Read the model definition and answer for the solid it produces. Units are mm, in the model's axes. Round coordinates to 2 decimals unless told otherwise and drop trailing zeros. Write each loop counter-clockwise with the first axis right and the second up, starting at its lowest first coordinate (ties: lowest second). Pieces come first, ordered by that corner, then holes.
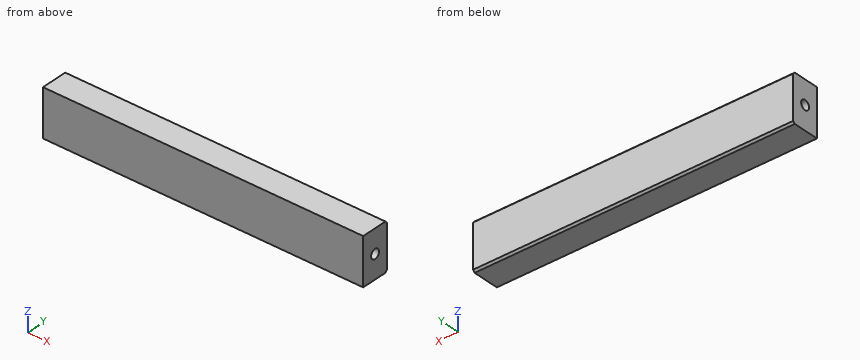
from build123d import *

# Parameters (mm, degrees)
SKETCH_1_W          = 85
SKETCH_1_H          = 7.5
EXTRUDE_1_DEPTH     = 12.5
SKETCH_2_R          = 1.25
CUT_EXTRUDE_1_DEPTH = 86.996002814
CHAMFER_1_SIZE      = 0.5


with BuildPart() as part:
    # 草图1 → 凸台-拉伸1 (new body)
    with BuildSketch(Plane.XY):
        Rectangle(SKETCH_1_W, SKETCH_1_H)
    extrude(amount=EXTRUDE_1_DEPTH)

    # 草图2 → 切除-拉伸1 (cut, through all)
    with BuildSketch(Plane(origin=(42.5, 0, 0), x_dir=(0, 0, -1), z_dir=(1, 0, 0))):
        with Locations((-6.25, 0)):
            Circle(SKETCH_2_R)
    extrude(amount=-CUT_EXTRUDE_1_DEPTH, mode=Mode.SUBTRACT)

    # 倒角1
    chamfer_1_edges = [part.edges().sort_by_distance(p)[0] for p in [
        (0, 3.75, 12.5),
        (0, 3.75, 0),
    ]]
    chamfer(chamfer_1_edges, length=CHAMFER_1_SIZE)


solid = part.part
Q1. Section A-A (z = 6.25) is taken. Determine the outline of the cut face in (x, y), then the cut area to 3 significant figures.
Verdict:
outline: (-42.5, -3.75) - (42.5, -3.75) - (42.5, -1.25) - (-42.5, -1.25) - close; (-42.5, 1.25) - (42.5, 1.25) - (42.5, 3.75) - (-42.5, 3.75) - close
area: 425 mm2
Q2. Section B-B (x = -6) is taken. Determine the outline of the cut face in (y, z), then the cut area to 3 significant figures.
Verdict:
outline: (-3.75, 0) - (3.25, 0) - (3.75, 0.5) - (3.75, 12) - (3.25, 12.5) - (-3.75, 12.5) - close; hole circle Ø2.5 at (0, 6.25)
area: 88.6 mm2
Q3. Straight lines are drawn through the part: probe 1 along Y at (x, z) = (15.5, 6.25); probe 2 along Z at (x, y) = (1, -0.25). For each, find the intervals that lie inside material, in ascending order.
Verdict:
probe 1: y = -3.75 to -1.25, 1.25 to 3.75
probe 2: z = 0 to 5.03, 7.47 to 12.5
Q4. Section C-C (y = 0) is taken. Determine the outline of the cut face in (x, z), then the cut area to 3 significant figures.
Verdict:
outline: (-42.5, 0) - (42.5, 0) - (42.5, 5) - (-42.5, 5) - close; (-42.5, 7.5) - (42.5, 7.5) - (42.5, 12.5) - (-42.5, 12.5) - close
area: 850 mm2
